Geometry: final body of the model. Coordinates: model frame, mm. Face numbers are marked on the shaded views. A direction names the side the tool comes from. Round coordinates to 2 decimals unless told otherwise and drop trailing zeros. Loops run counter-clockwise (first coordinate to the right, second up) from the corner with the lowest first, then second, coordinate; pieces in that order, holes last. Notation, with made-up numbers: (40.5, 4) - (48.5, 4) arc R12 ccw to (48.5, 17) - close; hole circle Ø2 at (-0.5, -2). An arc over 180 degrees is marked (long way). Answer as a JSON object with one key per item and string values. Group by question number.
Item 1: Section D-D (x = 43). Count the separate pieces of the cut face and the enclosed holes in it, plus the area to 3 significant figures.
Item 2: Draft query along Y for the marked faces 4, 5 and 6. Return one class per face: released by +Y, released by -Y, zero draft, split by the parting line, or undercut.
Item 3: Line query: line 1 (Y direction, x = -47.5, z = -18); line 2 (Y direction, x = -41, z = -20); line 3 (Y direction, x = 0, z = -22). Output: solid intervals per line, ascending.
Item 4: Section C-C (z = -35). Return the cut outline in (x, y).
Item 5: Reachability of the marked faces 1, 2 and 3 from +Z, -Z, +X, -X, +Y, -Y: full face, straight path, thin tool, end or side. Return the list, or none.
Item 6: First-contact query: pin 1 (1 mm diameter, centred on y = -17.5, z = -48.5, fed in from -X); pin 2 (12 mm diameter, centred on x = -47.5, y = 47.5, fed in from +Z); pin 3 (2 mm diameter, centred on y = -51, z = 10, fed in from -X); pin 4 (2 mm diameter, centred on y = -31, z = 20, fed in from -X). Flat tips, straight axial feed; report the tip coordinate or a pass-through.
Item 7: Section A-A (z = -20). Return the cut outline in (x, y), plus the area to 3 significant figures.
```python
from build123d import *

# Parameters (mm, degrees)
SKETCH1_R              = 55
BOSS_EXTRUDE1_DEPTH    = 30
SKETCH2_W              = 135
SKETCH2_H              = 135
BOSS_EXTRUDE2_DEPTH    = 40
SKETCH3_R              = 10
CUT_EXTRUDE1_DEPTH     = 40
SKETCH4_R              = 50
BOSS_EXTRUDE3_DEPTH    = 20
SKETCH5_R              = 45
BOSS_EXTRUDE4_DEPTH    = 5
SKETCH6_R              = 50
BOSS_EXTRUDE5_DEPTH    = 5
CHAMFER1_SIZE          = 2
CHAMFER2_SIZE          = 2
M20X2_5_TAPPED_HOLE1_D = 17.5
SKETCH9_R              = 35
CUT_EXTRUDE2_DEPTH     = 60
SKETCH10_R             = 30
CUT_EXTRUDE3_DEPTH     = 113.749722951


with BuildPart() as part:
    # Sketch1 → Boss-Extrude1 (new body)
    with BuildSketch(Plane.XY):
        Circle(SKETCH1_R)
    extrude(amount=BOSS_EXTRUDE1_DEPTH)

    # Sketch2 → Boss-Extrude2 (add)
    with BuildSketch(Plane(origin=(0, 0, 0), x_dir=(-1, 0, 0), z_dir=(0, 0, -1))):
        Rectangle(SKETCH2_W, SKETCH2_H)
    extrude(amount=BOSS_EXTRUDE2_DEPTH)

    # Sketch3 → Cut-Extrude1 (cut)
    with BuildSketch(Plane(origin=(0, 0, -40), x_dir=(-1, 0, 0), z_dir=(0, 0, -1))):
        with Locations((-47.5, 47.5)):
            Circle(SKETCH3_R)
        with Locations(Location((47.5, 47.5, 0), (0, 0, 180))):
            Circle(SKETCH3_R)
        with Locations((47.5, -47.5)):
            Circle(SKETCH3_R)
        with Locations(Location((-47.5, -47.5, 0), (0, 0, 180))):
            Circle(SKETCH3_R)
    extrude(amount=-CUT_EXTRUDE1_DEPTH, mode=Mode.SUBTRACT)

    # Sketch4 → Boss-Extrude3 (add)
    with BuildSketch(Plane(origin=(0, 0, -40), x_dir=(-1, 0, 0), z_dir=(0, 0, -1))):
        Circle(SKETCH4_R)
    extrude(amount=BOSS_EXTRUDE3_DEPTH)

    # Sketch5 → Boss-Extrude4 (add)
    with BuildSketch(Plane(origin=(0, 0, -60), x_dir=(-1, 0, 0), z_dir=(0, 0, -1))):
        Circle(SKETCH5_R)
    extrude(amount=BOSS_EXTRUDE4_DEPTH)

    # Sketch6 → Boss-Extrude5 (add)
    with BuildSketch(Plane(origin=(0, 0, -65), x_dir=(-1, 0, 0), z_dir=(0, 0, -1))):
        Circle(SKETCH6_R)
    extrude(amount=BOSS_EXTRUDE5_DEPTH)

    # Chamfer1
    chamfer1_edges = [part.edges().sort_by_distance(p)[0] for p in [
        (-55, 0, 30),
    ]]
    chamfer(chamfer1_edges, length=CHAMFER1_SIZE)

    # Chamfer2
    chamfer2_edges = [part.edges().sort_by_distance(p)[0] for p in [
        (50, 0, -70),
    ]]
    chamfer(chamfer2_edges, length=CHAMFER2_SIZE)

    # M20x2.5 Tapped Hole1 (through all)
    with Locations(Plane.ZY.offset(67.5)):
        with Locations((-20, 0)):
            Hole(M20X2_5_TAPPED_HOLE1_D / 2)

    # Sketch9 → Cut-Extrude2 (cut)
    with BuildSketch(Plane(origin=(0, 0, -70), x_dir=(-1, 0, 0), z_dir=(0, 0, -1))):
        Circle(SKETCH9_R)
    extrude(amount=-CUT_EXTRUDE2_DEPTH, mode=Mode.SUBTRACT)

    # Sketch10 → Cut-Extrude3 (cut, through all)
    with BuildSketch(Plane(origin=(0, 0, -10), x_dir=(-1, 0, 0), z_dir=(0, 0, -1))):
        Circle(SKETCH10_R)
    extrude(amount=-CUT_EXTRUDE3_DEPTH, mode=Mode.SUBTRACT)


solid = part.part
```
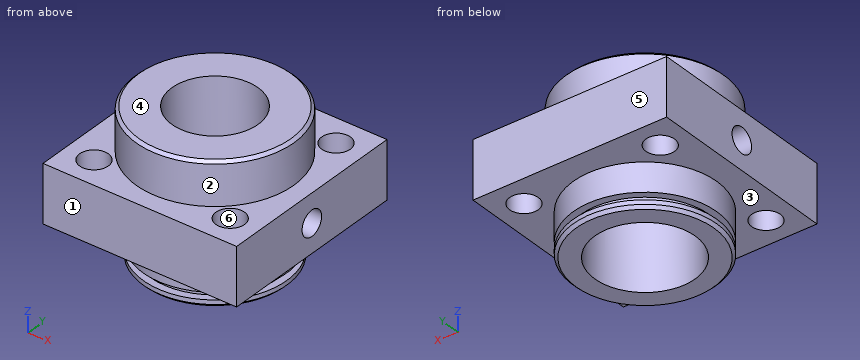
Values:
{
 "1": {"separate pieces": "3", "enclosed holes": "1", "area": "7,180 mm^2"},
 "2": {"face 4": "zero draft", "face 5": "released by +Y", "face 6": "undercut"},
 "3": {"line 1": "y = -67.5 to -57.5, -37.5 to -8.52, 8.52 to 37.5, 57.5 to 67.5", "line 2": "y = -67.5 to -55.1, -39.9 to -8.75, 8.75 to 39.9, 55.1 to 67.5", "line 3": "y = -67.5 to -35, 35 to 67.5"},
 "4": {"outline": "(-67.5, -67.5) - (67.5, -67.5) - (67.5, 67.5) - (-67.5, 67.5) - close; hole circle Ø20 at (-47.5, -47.5); hole circle Ø20 at (-47.5, 47.5); hole circle Ø70 at (0, 0); hole circle Ø20 at (47.5, -47.5); hole circle Ø20 at (47.5, 47.5)"},
 "5": {"face 1": "+Z, -Z, +X, -X, -Y", "face 2": "+Z", "face 3": "-Z"},
 "6": {"pin 1": "stops at x = -47.02", "pin 2": "passes through", "pin 3": "stops at x = -22.91", "pin 4": "stops at x = -46.1"},
 "7": {"outline": "(-67.5, -67.5) - (67.5, -67.5) - (67.5, -8.75) - (33.89, -8.75) arc R35 cw to (-33.89, -8.75) - (-67.5, -8.75) - close; (-67.5, 8.75) - (-33.89, 8.75) arc R35 cw to (33.89, 8.75) - (67.5, 8.75) - (67.5, 67.5) - (-67.5, 67.5) - close; hole circle Ø20 at (-47.5, -47.5); hole circle Ø20 at (-47.5, 47.5); hole circle Ø20 at (47.5, -47.5); hole circle Ø20 at (47.5, 47.5)", "area": "12,000 mm^2"}
}
